```python
from build123d import *

# Parameters (mm, degrees)
EXTRUDE_1_DEPTH                            = 3
SKETCH_2_W                                 = 139
SKETCH_2_H                                 = 47.74
CUT_EXTRUDE_1_DEPTH                        = 0.1
SKETCH_3_R                                 = 2.8
EXTRUDE_2_DEPTH                            = 4
SKETCH_4_R                                 = 1
CUT_EXTRUDE_2_DEPTH                        = 4
MIRROR_1_AT_THE_SECOND_PLANE_COPY_1_SKET_R = 2.8
MIRROR_1_AT_THE_SECOND_PLANE_COPY_1_DEPTH  = 4
MIRROR_1_AT_THE_SECOND_PLANE_COPY_2_SKET_R = 1
MIRROR_1_AT_THE_SECOND_PLANE_COPY_2_DEPTH  = 4
SKETCH_5_W                                 = 6
SKETCH_5_H                                 = 11
EXTRUDE_3_DEPTH                            = 1.7
SKETCH_6_W                                 = 6
SKETCH_6_H                                 = 17
EXTRUDE_4_DEPTH                            = 4


with BuildPart() as part:
    # ｽｹｯﾁ1 → ﾎﾞｽ - 押し出し1 (new body)
    with BuildSketch(Plane(origin=(0, 0, 0), x_dir=(1, 0, 0), z_dir=(0, 1, 0))):
        with BuildLine():
            Line((-75, 29.25), (75, 29.25))
            ThreePointArc((75, 29.25), (75.707106781, 28.957106781), (76, 28.25))
            Line((76, 28.25), (76, -28.25))
            ThreePointArc((76, -28.25), (75.707106781, -28.957106781), (75, -29.25))
            Line((75, -29.25), (-75, -29.25))
            ThreePointArc((-75, -29.25), (-75.707106781, -28.957106781), (-76, -28.25))
            Line((-76, -28.25), (-76, 28.25))
            ThreePointArc((-76, 28.25), (-75.707106781, 28.957106781), (-75, 29.25))
        make_face()
    extrude(amount=EXTRUDE_1_DEPTH)

    # ｽｹｯﾁ2 → ｶｯﾄ - 押し出し1 (cut)
    with BuildSketch(Plane(origin=(0, 3, 0), x_dir=(1, 0, 0), z_dir=(0, 1, 0))):
        with Locations((4, 0)):
            Rectangle(SKETCH_2_W, SKETCH_2_H)
    extrude(amount=-CUT_EXTRUDE_1_DEPTH, mode=Mode.SUBTRACT)

    # ｽｹｯﾁ3 → ﾎﾞｽ - 押し出し2 (add)
    with BuildSketch(Plane.XZ):
        with Locations(Location((-71.5, 24.75, 0), (0, 0, 270))):
            Circle(SKETCH_3_R)
    extrude_2 = extrude(amount=EXTRUDE_2_DEPTH)

    # ｽｹｯﾁ4 → ｶｯﾄ - 押し出し2 (cut)
    with BuildSketch(Plane.XZ.offset(4)):
        with Locations(Location((-71.5, 24.75, 0), (0, 0, 270))):
            Circle(SKETCH_4_R)
    cut_extrude_2 = extrude(amount=-CUT_EXTRUDE_2_DEPTH, mode=Mode.SUBTRACT)

    # ﾐﾗｰ1: ﾎﾞｽ - 押し出し2, ｶｯﾄ - 押し出し2 across plane
    add(extrude_2.mirror(Plane(origin=(0, 0, 0), x_dir=(0, 0, 1), z_dir=(1, 0, 0))))
    add(cut_extrude_2.mirror(Plane(origin=(0, 0, 0), x_dir=(0, 0, 1), z_dir=(1, 0, 0))), mode=Mode.SUBTRACT)

    # ﾐﾗｰ1 at the second plane: ﾎﾞｽ - 押し出し2, ｶｯﾄ - 押し出し2 across plane
    add(extrude_2.mirror(Plane.XY))
    add(cut_extrude_2.mirror(Plane.XY), mode=Mode.SUBTRACT)

    # ﾐﾗｰ1 at the second plane copy 1 sket → ﾐﾗｰ1 at the second plane copy 1 (add)
    with BuildSketch(Plane(origin=(0, 0, 0), x_dir=(-1, 0, 0), z_dir=(0, -1, 0))):
        with Locations(Location((-71.5, 24.75, 0), (0, 0, 270))):
            Circle(MIRROR_1_AT_THE_SECOND_PLANE_COPY_1_SKET_R)
    extrude(amount=MIRROR_1_AT_THE_SECOND_PLANE_COPY_1_DEPTH)

    # ﾐﾗｰ1 at the second plane copy 2 sket → ﾐﾗｰ1 at the second plane copy 2 (cut)
    with BuildSketch(Plane(origin=(0, -4, 0), x_dir=(-1, 0, 0), z_dir=(0, -1, 0))):
        with Locations(Location((-71.5, 24.75, 0), (0, 0, 270))):
            Circle(MIRROR_1_AT_THE_SECOND_PLANE_COPY_2_SKET_R)
    extrude(amount=-MIRROR_1_AT_THE_SECOND_PLANE_COPY_2_DEPTH, mode=Mode.SUBTRACT)

    # ｽｹｯﾁ5 → ﾎﾞｽ - 押し出し3 (add)
    with BuildSketch(Plane.XZ):
        with Locations((-60, 0)):
            Rectangle(SKETCH_5_W, SKETCH_5_H)
    extrude(amount=EXTRUDE_3_DEPTH)

    # ｽｹｯﾁ6 → ﾎﾞｽ - 押し出し4 (add)
    with BuildSketch(Plane.XZ):
        with Locations((64.5, 0)):
            Rectangle(SKETCH_6_W, SKETCH_6_H)
    extrude(amount=EXTRUDE_4_DEPTH)


solid = part.part
```
Model file for the job. Use its own axes, mm. A direction names the side the tool comes from. Round coordinates to 2 decimals unless told otherwise and drop trailing zeros. Order: outer loops, then holes, each group sorted by start corner. A loop starts at its lowest first (then second) coordinate and runs counter-clockwise, first axis right, second up. Notation, with made-up numbers: (-27.75, 40) -> (-19.75, 40) arc R23 cw to (-19.75, 73) -> close; hole circle Ø5 at (66, 84). An arc over 180 degrees is marked (long way). Use one line per item in the form item = value.
Item 1: Cut at C-C, the plane z = 7. Write the cut outline in (x, y), and give its area (3 significant figures).
Returned:
outline = (-76, 0) -> (61.5, 0) -> (61.5, -4) -> (67.5, -4) -> (67.5, 0) -> (76, 0) -> (76, 3) -> (73.5, 3) -> (73.5, 2.9) -> (-65.5, 2.9) -> (-65.5, 3) -> (-76, 3) -> close
area = 466 mm^2
Item 2: Drill centre lines: line 1 (X direction, y = -2.05, z = 24.75); line 2 (Z direction, x = 71.5, y = -1.5); line 3 (X direction, y = -1.5, z = 2). Where is each one in solid material? Low to high.
Returned:
line_1 = -74.3 to -72.5, -70.5 to -68.7, 68.7 to 70.5, 72.5 to 74.3
line_2 = -27.55 to -25.75, -23.75 to -21.95, 21.95 to 23.75, 25.75 to 27.55
line_3 = -63 to -57, 61.5 to 67.5
Item 3: Pull direction Z, two halves, no side cores. Call faces 6 (the face through (64, -4, 0)), 7 (the face through (1, 1, 29.25)), 8 (the face through (-68.724, -1.972, 25.115)): released by +Z, released by -Z, zero draft, split by the parting line, or undercut.
Returned:
face_6 = zero draft
face_7 = released by +Z
face_8 = undercut
Item 4: Cut at A-A, the plane z = -1. Write the cut outline in (x, y).
Returned:
outline = (-76, 0) -> (-63, 0) -> (-63, -1.7) -> (-57, -1.7) -> (-57, 0) -> (61.5, 0) -> (61.5, -4) -> (67.5, -4) -> (67.5, 0) -> (76, 0) -> (76, 3) -> (73.5, 3) -> (73.5, 2.9) -> (-65.5, 2.9) -> (-65.5, 3) -> (-76, 3) -> close
Item 5: Flat gauge pins, fed straight in: pin 1 Ø4 at (x, z) = (59, -7) entering from +Y; pin 2 Ø1.2 at (y, z) = (-2.5, 4) entering from -X; pin 3 Ø3 at (x, y) = (65, -2.5) entering from +Z. Where does each tip first touch, or does it go through?
Returned:
pin_1 = 2.9
pin_2 = 61.5
pin_3 = 8.5
Item 6: Tool access for faces 1 (the face through (61.5, -2, 0)), 2 (the face through (68.724, -1.972, -25.115)), 3 (the face through (-60, -1.7, 0)), 4 (the face through (64, -2, -8.5)), 5 (the face through (3, 2.9, 0)): list every direction of +Z, -Z, +X, -X, +Y, -Y with a clear straight run to the whole face (end or side of a thin tool).
Returned:
face_1 = +Z, -Z, -Y
face_2 = -Y
face_3 = +Z, -Z, -X, -Y
face_4 = -Z, +X, -X, -Y
face_5 = +Y
Item 7: Cut at B-B, the plane x = 4. Write the cut outline in (y, z).
Returned:
outline = (0, -29.25) -> (3, -29.25) -> (3, -23.87) -> (2.9, -23.87) -> (2.9, 23.87) -> (3, 23.87) -> (3, 29.25) -> (0, 29.25) -> close
